Check sheet for the modelled part. Datum: model origin and axes. Units: mm. Face numbers are marked on the shaded views. A direction names the side the tool comes from. Give positions to 0.01 mm unless a question says otherwise; leave off trailing zeros. Loops run counter-clockwise (first coordinate to the right, second up) from the corner with the lowest first, then second, coordinate; pieces in that order, holes last. Notation, with made-up numbers: M 0.5,-9 L 41.5,-9 A19 cw 41.5,3 Z; hole C 43,85 d7. An arc over 180 degrees is marked long. One line per question, with ' | ' between items. Start each with the question number.
from build123d import *

# Parameters (mm, degrees)
SKETCH_1_R          = 1.525
EXTRUDE_1_DEPTH     = 2
FILLET_1_R          = 2
SKETCH_3_R          = 2.525
CUT_EXTRUDE_1_DEPTH = 11
SKETCH_4_R          = 2.025
CUT_EXTRUDE_2_DEPTH = 20
CUT_EXTRUDE_3_DEPTH = 20
FILLET_2_R          = 1.5
CUT_EXTRUDE_4_DEPTH = 10
EXTRUDE_2_DEPTH     = 4
FILLET_3_R          = 1.5


with BuildPart() as part:
    # 草图1 → 凸台-拉伸1 (new, symmetric)
    with BuildSketch(Plane.XY):
        with BuildLine():
            Line((-14, -25), (14, -25))
            Line((14, -25), (14, 25))
            ThreePointArc((14, 25), (16.980954382, 43.334686237), (25.616740047, 59.780658824))
            ThreePointArc((25.616740047, 59.780658824), (25.857254614, 64.865842734), (21.215464165, 66.956470411))
            ThreePointArc((21.215464165, 66.956470411), (-4.029350016, 52.38829278), (-14, 25))
            Line((-14, 25), (-14, -25))
        make_face()
        with Locations((22, 62.5)):
            Circle(SKETCH_1_R, mode=Mode.SUBTRACT)
    extrude(amount=EXTRUDE_1_DEPTH, both=True)

    # 圆角1
    fillet_1_edges = [part.edges().sort_by_distance(p)[0] for p in [
        (14, -25, 0),
        (-14, -25, 0),
    ]]
    fillet(fillet_1_edges, radius=FILLET_1_R)

    # 草图3 → 切除-拉伸1 (cut, symmetric)
    with BuildSketch(Plane.XY.offset(2)):
        with Locations(Location((22, 62.5, 0), (0, 0, 180))):
            Circle(SKETCH_3_R)
    extrude(amount=CUT_EXTRUDE_1_DEPTH, both=True, mode=Mode.SUBTRACT)

    # 草图4 → 切除-拉伸2 (cut)
    with BuildSketch(Plane.XY.offset(2)):
        with Locations((-10.004554112, 9.95)):
            Circle(SKETCH_4_R)
        with Locations((9.995445888, 9.95)):
            Circle(SKETCH_4_R)
        with Locations((9.995445888, -19.95)):
            Circle(SKETCH_4_R)
        with Locations((-10.004554112, -19.95)):
            Circle(SKETCH_4_R)
    extrude(amount=-CUT_EXTRUDE_2_DEPTH, mode=Mode.SUBTRACT)

    # 草图5 → 切除-拉伸3 (cut)
    with BuildSketch(Plane.XY.offset(2)):
        with BuildLine():
            ThreePointArc((-10.004554112, -14.95), (-6.469020206, -16.414466094), (-5.004554112, -19.95))
            Line((-5.004554112, -19.95), (4.995445888, -19.95))
            ThreePointArc((4.995445888, -19.95), (6.459911982, -16.414466094), (9.995445888, -14.95))
            Line((9.995445888, -14.95), (9.995445888, 4.95))
            ThreePointArc((9.995445888, 4.95), (6.459911982, 6.414466094), (4.995445888, 9.95))
            Line((4.995445888, 9.95), (-5.004554112, 9.95))
            ThreePointArc((-5.004554112, 9.95), (-6.469020206, 6.414466094), (-10.004554112, 4.95))
            Line((-10.004554112, 4.95), (-10.004554112, -14.95))
        make_face()
    extrude(amount=-CUT_EXTRUDE_3_DEPTH, mode=Mode.SUBTRACT)

    # 圆角2
    fillet_2_edges = [part.edges().sort_by_distance(p)[0] for p in [
        (9.995445888, -14.95, 0),
        (4.995445888, -19.95, 0),
        (-5.004554112, -19.95, 0),
        (-10.004554112, -14.95, 0),
        (-10.004554112, 4.95, 0),
        (-5.004554112, 9.95, 0),
        (4.995445888, 9.95, 0),
        (9.995445888, 4.95, 0),
    ]]
    fillet(fillet_2_edges, radius=FILLET_2_R)

    # 草图6 → 切除-拉伸4 (cut)
    with BuildSketch(Plane.XY.offset(2)):
        with BuildLine():
            Line((-9, 25), (-9, 16.95))
            Line((-9, 16.95), (9, 16.95))
            Line((9, 16.95), (9, 25))
            ThreePointArc((9, 25), (11.284284207, 41.793802743), (17.971158754, 57.367353196))
            ThreePointArc((17.971158754, 57.367353196), (16.686132643, 58.713386908), (15.833336193, 60.367423509))
            ThreePointArc((15.833336193, 60.367423509), (-2.171664491, 46.607575246), (-9, 25))
        make_face()
    extrude(amount=-CUT_EXTRUDE_4_DEPTH, mode=Mode.SUBTRACT)

    # 草图7 → 凸台-拉伸2 (add)
    with BuildSketch(Plane.XY.offset(2)):
        Polygon((-4.043281882, 45.902558691), (7.128382609, 16.244983445), (10.871617391, 17.655016555), (-0.748810192, 48.503929507), align=None)
    extrude(amount=-EXTRUDE_2_DEPTH)

    # 圆角3
    fillet_3_edges = [part.edges().sort_by_distance(p)[0] for p in [
        (-0.748810192, 48.503929507, 0),
        (15.833336193, 60.367423509, 0),
        (9, 22.623625632, 0),
        (17.971158754, 57.367353196, 0),
        (-3.527808844, 44.534125149, 0),
        (-9, 16.95, 0),
        (6.862811053, 16.95, 0),
    ]]
    fillet(fillet_3_edges, radius=FILLET_3_R)


solid = part.part
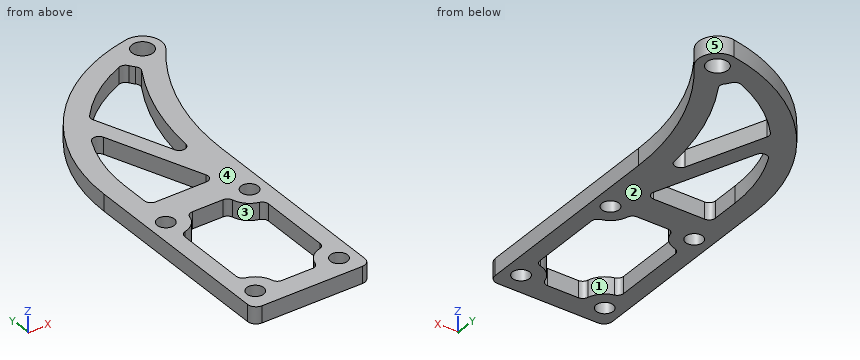
Q1. Cross-section at B-B (x = 1.5). Record the cut outline in (y, z).
Q2. Draft check along Y on the marked faces 3, 4 and 5. Enter one of: released by +Y, released by -Y, zero draft, split by the parting line, or undercut.
Q3. Depth check by flat-ended pin: P1, Ø1, axis at x = -1, z = 1, coming from the +Y side; P2, Ø1.2, axis at x = 0, z = 0, coming from the +Y side; P3, Ø2, axis at y = 21.5, z = 1, coming from the +X side. Enter the tip coordinate at first touch or a pass-through.
Q4. Cross-section at D-D (z = 1.1). State how many separate pieces and enclosed holes the cut face has, and give its area (3 significant figures).
Q5. Access from +Z, -Z, +X, -X, +Y, -Y to the whole of each face (thin tool, end or side, straight path). Record for the marked faces 1 and 2.
Q6. Cross-section at A-A (y = 20). Record the cut outline in (x, z), and give its area (3 significant figures).
Q7. Material ranges on probe 1 along X at (y, z) = (-13, 1.05); probe 2 along Y at (x, z) = (-9.5, 1.1); probe 3 along X at (y, z) = (61.5, 1.6), recorded low to high. Write a range as from..to.
Q8. Cross-section at C-C (y = -1.5). Record the cut outline in (x, z), and give its area (3 significant figures).
Solved:
1) outline: M -25,-2 L -19.95,-2 L -19.95,2 L -25,2 Z; M 9.95,-2 L 16.95,-2 L 16.95,2 L 9.95,2 Z; M 31.19,-2 L 42.53,-2 L 42.53,2 L 31.19,2 Z; M 51.07,-2 L 57.87,-2 L 57.87,2 L 51.07,2 Z
2) face 3: undercut | face 4: zero draft | face 5: split by the parting line
3) P1: stops at y = 56.11 | P2: stops at y = 57.11 | P3: stops at x = 14
4) separate pieces: 1 | enclosed holes: 8 | area: 1,310 mm²
5) face 1: +Z, -Z | face 2: -Z, +X, -X, +Y, -Y
6) outline: M -14,-2 L -9,-2 L -9,2 L -14,2 Z; M 5.71,-2 L 14,-2 L 14,2 L 5.71,2 Z | area: 53.1 mm²
7) probe 1: x = -14..-10, 10..14 | probe 2: y = -25..-21.91, -17.99..-14.75, 4.75..7.99, 11.91..44.06 | probe 3: x = 6.63..19.68, 24.32..26.41
8) outline: M -14,-2 L -10,-2 L -10,2 L -14,2 Z; M 10,-2 L 14,-2 L 14,2 L 10,2 Z | area: 32.0 mm²
